```python
from build123d import *

# Parameters (mm, degrees)
SKETCH3_R           = 1.190625
BOSS_EXTRUDE1_DEPTH = 1.5875


with BuildPart() as part:
    # Sketch3 → Boss-Extrude1 (new body)
    with BuildSketch(Plane(origin=(0, 0, 0), x_dir=(1, 0, 0), z_dir=(0, 1, 0))):
        Polygon((-22.929311402, 25.613223092), (-13.634997975, 33.054629342), (20.099377025, 33.054629342), (29.393690453, 25.613223092), (34.156190453, 31.968309197), (24.861877025, 39.409715447), (20.902655838, 42.579629342), (-14.438276788, 42.579629342), (-18.397497975, 39.409715447), (-27.691811402, 31.968309197), align=None)
        with Locations(Location((-19.770435938, 31.192788903, 0), (0, 0, 270))):
            Circle(SKETCH3_R, mode=Mode.SUBTRACT)
        with Locations(Location((26.234814989, 31.192788903, 0), (0, 0, 270))):
            Circle(SKETCH3_R, mode=Mode.SUBTRACT)
    extrude(amount=BOSS_EXTRUDE1_DEPTH)

    # Fillet1
    # a fillet whose section is not a circle: 3.175 mm, written as the material it takes off along each edge
    with BuildSketch(Plane(origin=(-22.929311402, -8.195772914, -25.613223092), x_dir=(0.7806247497998012, 0, -0.6249999999999982), z_dir=(0, 1, 0)), Plane(origin=(29.393690453, -8.195772914, -25.613223092), x_dir=(0.5996925441644039, 0, -0.8002304995897274), z_dir=(0, 1, 0))) as fillet1_piece_1:
        with BuildLine():
            Bezier((3.278309166, 0), (0, 0), (0.104936119, 3.276629273), weights=[1, 0.448951306, 1])
            Line((0.104936119, 3.276629273), (0, 0))
            Line((0, 0), (3.278309166, 0))
        make_face()
    extrude(amount=17.979045828, mode=Mode.SUBTRACT)
    with BuildSketch(Plane(origin=(-27.691811402, -7.687366025, -31.968309197), x_dir=(0.7806247497998011, 0, -0.6249999999999983), z_dir=(0, 1, 0))) as fillet1_piece_2:
        with BuildLine():
            Bezier((3.07494641, 0), (0, 0), (-0.098426636, -3.073370727), weights=[1, 0.463559427, 1])
            Line((-0.098426636, -3.073370727), (0, 0))
            Line((0, 0), (3.07494641, 0))
        make_face()
    extrude(amount=16.962232051, mode=Mode.SUBTRACT)
    with BuildSketch(Plane(origin=(34.156190453, -7.687366025, -31.968309197), x_dir=(-0.7806247497995835, 0, -0.62500000000027), z_dir=(0, 1, 0))) as fillet1_piece_3:
        with BuildLine():
            Bezier((3.07494641, 0), (0, 0), (-0.098426636, 3.073370727), weights=[1, 0.463559427, 1])
            Line((-0.098426636, 3.073370727), (0, 0))
            Line((0, 0), (3.07494641, 0))
        make_face()
    extrude(amount=16.962232051, mode=Mode.SUBTRACT)
    with BuildSketch(Plane(origin=(20.902655838, -2.786065678, -42.579629342), x_dir=(-1, 0, 0), z_dir=(0, 1, 0)), Plane(origin=(-14.438276788, -2.786065678, -42.579629342), x_dir=(-0.780624749799802, 0, 0.6249999999999972), z_dir=(0, 1, 0))) as fillet1_piece_4:
        with BuildLine():
            Bezier((1.114426271, 0), (0, 0), (-0.869948729, 0.696516419), weights=[1, 0.608905409, 1])
            Line((-0.869948729, 0.696516419), (0, 0))
            Line((0, 0), (1.114426271, 0))
        make_face()
    extrude(amount=7.159631355, mode=Mode.SUBTRACT)


solid = part.part
```
Here's how the part is built. I have some questions about the finished solid (model axes, mm). A direction names the side the tool comes from. Round coordinates to 2 decimals unless told otherwise and drop trailing zeros. Order: outer loops, then holes, each group sorted by start corner. A loop starts at its lowest first (then second) coordinate and runs counter-clockwise, first axis right, second up. Notation, with made-up numbers: M 0,62 L 52,62 A21 cw 52,84 Z; hole C 3.25,43.25 d1. An arc over 180 degrees is marked long. Answer in a Markdown table with one row per item.
Item 1: I'm going to push a flat-ended pin straight in: pin 1 (3 mm diameter, centred on x = -12.5, z = -30.5, fed in from +Y). Where does the tip first touch, or does it pass through?
A:
| item | result |
|---|---|
| pin 1 | passes through |
Item 2: Thinking about a two-plate mould opening in X: for faces 1 (the face through (3, 0, -37)), 2 (the face through (31.829, 0.783, -28.863)), 3 (the face through (-19.718, 0.783, -32.382)), which applies, +X half, -X half, draft (parallel to the pull), parting line (faces both ways), or undercut?
A:
| item | result |
|---|---|
| face 1 | draft |
| face 2 | +X half |
| face 3 | undercut |
Item 3: Imagine slicing it at C-C, the plane z = -36. Write out the boundary of the cut face in (x, y).
A:
| item | result |
|---|---|
| outline | M -22.66,0 L 29.12,0 L 29.12,1.59 L -22.66,1.59 Z |
Item 4: For faces 4 (the face through (25.073, 0.783, -31.451)), 5 (the face through (23.42, 0.783, -30.396)), which set-ups out of +Z, -Z, +X, -X, +Y, -Y let a thin tool reach every point of the face, with its end or its side?
A:
| item | result |
|---|---|
| face 4 | +Y, -Y |
| face 5 | +Z, +Y, -Y |
Item 5: Imagine slicing it at A-A, the plane z = -31. State how many separate pieces and enclosed holes the cut face has, and give its area (3 significant figures).
A:
| item | result |
|---|---|
| separate pieces | 4 |
| enclosed holes | 0 |
| area | 24.5 mm2 |
Item 6: Imagine slicing it at B-B, the plane x = -11.5. Write out the boundary of the cut face in (y, z).
A:
| item | result |
|---|---|
| outline | M 0,-42.58 L 1.59,-42.58 L 1.59,-33.05 L 0,-33.05 Z |
Item 7: If I drill on L1, parallel to X at y = 0.9, z = -30.25 (3 decimals); L2, parallel to Z at x = 7, y = 0.9; L3, parallel to X at y = 1, z = -32, over which ranges is the centre line in solid material (lowest first)? Write a range as from..to.
A:
| item | result |
|---|---|
| L1 | x = -26.175..-20.498, -19.043..-17.138, 23.602..25.508, 26.962..32.639 |
| L2 | z = -42.58..-33.05 |
| L3 | x = -26.21..-20.65, -18.9..-14.95, 21.42..25.36, 27.11..32.67 |
